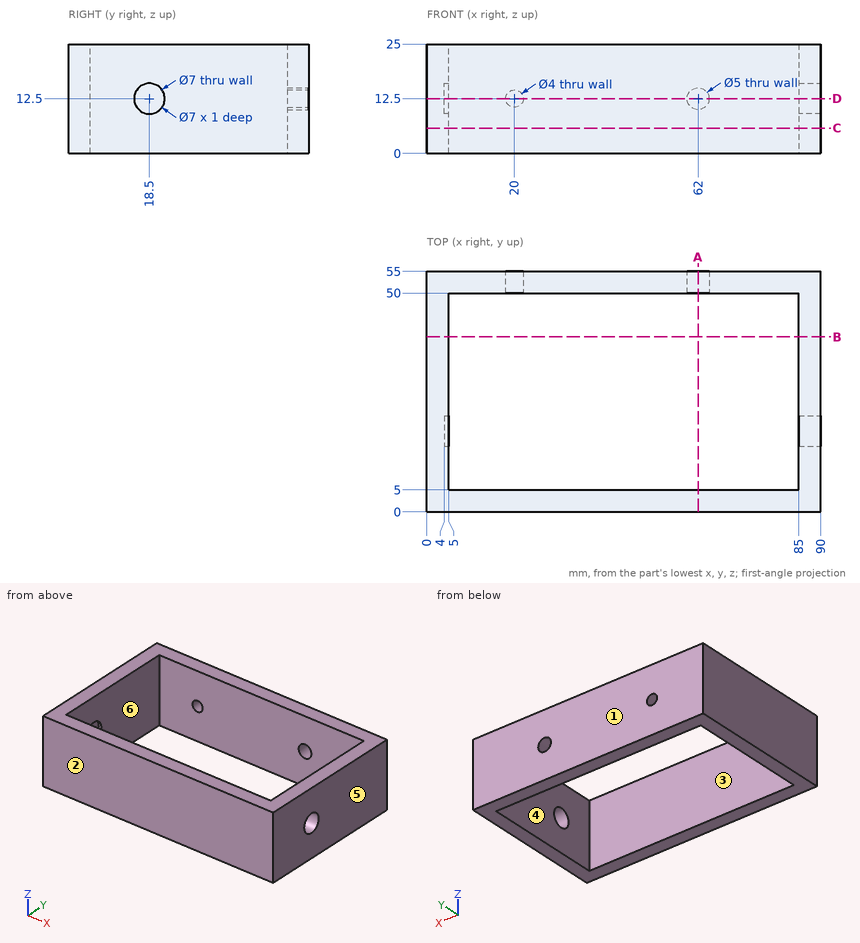
Job drawing, mm, ordinate dimensions from the low corner. One solid piece. A direction names the side the tool comes from. Coordinates: 2 decimals unless noted, no trailing zeros. Order: outer loops, then holes, each group sorted by start corner. A loop starts at its lowest first (then second) coordinate and runs counter-clockwise, first axis right, second up. Notation, with made-up numbers: (25.25, -35.75) -> (75.25, -35.75) arc R31 ccw to (75.25, -7.75) -> close; hole circle Ø3 at (22.5, 51.25). An arc over 180 degrees is marked (long way). Put each result on its own line as item: value. Start each with the question number.
(1) Band-saw the part on D-D (z = 12.5). Give the cut face in (x, y), then the cut area to 3 significant figures.
(2) Which spindle directions (+Z, -Z, +X, -X, +Y, -Y) get a long thin tool onto all of the face, cutting with end or side? Do the marked faces 5 and 6. Say none if no direction does.
(3) Band-saw the part on C-C (z = 5.75). Give the cut face in (x, y), then the cut area to 3 significant figures.
(4) Pin check, flat tips, straight feed: pin 1 Ø2.5 at (x, z) = (20, 12.5) entering from +Y; pin 2 Ø6.5 at (y, z) = (18.5, 12.5) entering from +X. Stop position of each tip, or through.
(5) Probe line 1 along Y through (x, z) = (26.5, 5.25); line 2 along X through (y, z) = (10.5, 1.5); line 3 along X through (y, z) = (53.1, 12.5). List the from-to ranges inside material, lowest first. Write a range as [from, to].
(6) Band-saw the part on B-B (y = 40). Give the cut face in (x, z).
(7) Band-saw the part on A-A (x = 62). Give the cut face in (y, z), then the cut area to 3 significant figures.
(8) Mould opens along Y. For the marked faces 1, 2, 3 and 4 say: pulls with the +Y half, pulls with the -Y half, needs draft (parallel to the pull), parting line crosses it, or undercut.
Determined:
1. outline: (0, 0) -> (90, 0) -> (90, 15) -> (85, 15) -> (85, 5) -> (5, 5) -> (5, 15) -> (4, 15) -> (4, 22) -> (5, 22) -> (5, 50) -> (18, 50) -> (18, 55) -> (0, 55) -> close; (22, 50) -> (59.5, 50) -> (59.5, 55) -> (22, 55) -> close; (64.5, 50) -> (85, 50) -> (85, 22) -> (90, 22) -> (90, 55) -> (64.5, 55) -> close
1. area: 1,260 mm²
2. face 5: +Z, -Z, +X, +Y, -Y
2. face 6: +Z, -Z
3. outline: (0, 0) -> (90, 0) -> (90, 55) -> (0, 55) -> close; hole (5, 5) -> (85, 5) -> (85, 50) -> (5, 50) -> close
3. area: 1,350 mm²
4. pin 1: stops at y = 5
4. pin 2: stops at x = 4
5. line 1: y = [0, 5], [50, 55]
5. line 2: x = [0, 5], [85, 90]
5. line 3: x = [0, 18], [22, 59.5], [64.5, 90]
6. outline: (0, 0) -> (5, 0) -> (5, 25) -> (0, 25) -> close; (85, 0) -> (90, 0) -> (90, 25) -> (85, 25) -> close
7. outline: (0, 0) -> (5, 0) -> (5, 25) -> (0, 25) -> close; (50, 0) -> (55, 0) -> (55, 10) -> (50, 10) -> close; (50, 15) -> (55, 15) -> (55, 25) -> (50, 25) -> close
7. area: 225 mm²
8. face 1: pulls with the +Y half
8. face 2: pulls with the -Y half
8. face 3: undercut
8. face 4: undercut
